Solid Edge part; units mm, degrees
sketch "Sketch1" plane through (0, 0, 0) normal (0, -1, 0) x (1, 0, 0)
  line L0 (0, 0) -> (0, -330.2)
  line L1 (0, 0) -> (0, 330.2)
  arc A0 (0, 330.2) -> (0, -330.2) centre (0, 0) cw
revolve "RevolvedProtrusion1" add sketch "Sketch1" angle 360 about axis through (0, 0, 0) along (0, 0, 1)
sketch "Sketch2" plane through (0, 0, 0) normal (0, -1, 0) x (1, 0, 0)
  line L0 (0, -305.264) -> (125.8807, -305.264)
revolve "RevolvedCutout1" cut sketch "Sketch2" angle 360 about axis through (0, 0, -305.264) along (0, 0, -1) material side at (62.9404, 0, -305.314)
sketch "Sketch3" plane through (0, 0, 0) normal (0, -1, 0) x (1, 0, 0)
  line L0 (0, -76.2) -> (330.2, -76.2)
  line L1 (330.2, 0) -> (330.2, -76.2)
  line L2 (0, 0) -> (330.2, 0)
  line L3 (0, 0) -> (0, -76.2)
revolve "RevolvedProtrusion2" add sketch "Sketch3" angle 360 about axis through (0, 0, 0) along (0, 0, -1)
sketch "Sketch4" plane through (0, 0, 330.2) normal (0, 0, 1) x (1, 0, 0)
  circle A0 centre (0, 0) radius 25.4
extrude "Protrusion1" add sketch "Sketch4" against normal up to vertex (330.2 mm away) and the other way blind 25.4
shell "Thinwall_1" thickness 6.35 removed faces 1 at (-17.4413, -16.4253, 355.6)
sketch "Sketch5" plane through (0, 0, 355.6) normal (0, 0, 1) x (0, -1, 0)
  circle A0 centre (0, 0) radius 19.05
  circle A1 centre (0, 0) radius 6.35
extrude "ExtrudedProtrusion_3" add sketch "Sketch5" against normal blind 6.35
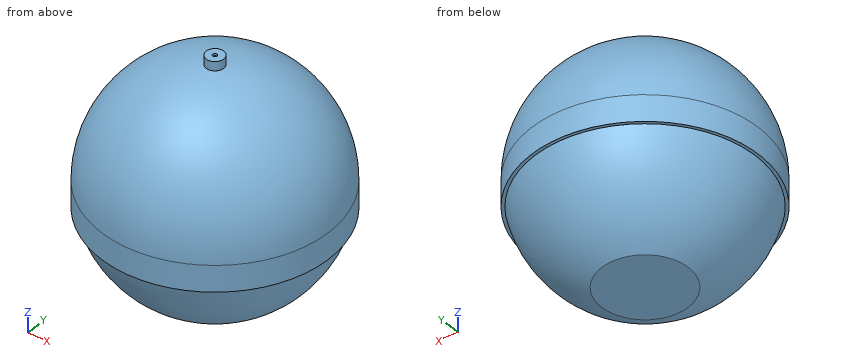
Source: CAD feature listing. Evaluate the final solid. Frame: model axes, mm. Give positions to 0.01 mm unless a question says otherwise; leave off trailing zeros. Write each loop counter-clockwise with the first axis right and the second up, starting at its lowest first coordinate (ties: lowest second). Pieces come first, ordered by that corner, then holes. Notation, with made-up numbers: (35.25, 67.5) - (72.25, 67.5) arc R21 cw to (72.25, 99.5) - close; hole circle Ø8 at (-17.5, -39). An arc over 180 degrees is marked (long way). One line per item, written item: value. Start each with the question number.
Q1. Section query D-D, the plane y = -112.5. Return the cut outline in (x, z), then the cut area to 3 significant figures.
Q2. Section query A-A, the plane y = 277. Return the cut outline in (x, z), then the cut area to 3 significant figures.
Q3. First-contact query: pin 1 Ø4 at (x, y) = (-200.5, 0) entering from -Z; pin 2 Ø6 at (y, z) = (-13.5, -40.5) entering from +X; pin 3 Ø2 at (y, z) = (-105.5, 99.5) entering from +X. Flat tips, straight axial feed; report the tip coordinate or a pass-through.
Q4. Material intervals for probe 1 along Y at (x, z) = (0, 331); probe 2 along X at (y, z) = (129.5, 67.5); probe 3 along X at (y, z) = (-111, -8), sorted ascending. Write a range as from..to.
Q5. Section query B-B, the plane x = -286.5. Return the cut outline in (y, z).
Q6. Section query C-C, the plane z = -46.5. Return the cut outline in (x, y).
Answer:
1. outline: (-310.44, -76.2) - (-300.95, -76.2) arc R310.44 ccw to (-56.48, -305.26) - (56.48, -305.26) arc R310.44 ccw to (300.95, -76.2) - (310.44, -76.2) - (310.44, 0) arc R310.44 ccw to (-310.44, 0) - close; hole (-303.68, -69.85) - (-295.54, -69.85) arc R303.68 ccw to (-53.6, -298.91) - (53.6, -298.91) arc R303.68 ccw to (295.54, -69.85) - (303.68, -69.85) - (303.68, 0) arc R303.68 ccw to (-303.68, 0) - close
1. area: 13,100 mm2
2. outline: (-179.73, -76.2) - (-162.78, -76.2) arc R179.73 ccw to (162.78, -76.2) - (179.73, -76.2) - (179.73, 0) arc R179.73 ccw to (-179.73, 0) - close; hole (-167.78, -69.85) - (-152.55, -69.85) arc R167.78 ccw to (152.55, -69.85) - (167.78, -69.85) - (167.78, 0) arc R167.78 ccw to (-167.78, 0) - close
2. area: 13,200 mm2
3. pin 1: stops at z = -263.87
3. pin 2: stops at x = 330.03
3. pin 3: stops at x = 297.14
4. probe 1: y = -25.4..-19.05, 19.05..25.4
4. probe 2: x = -296.15..-289.05, 289.05..296.15
4. probe 3: x = -310.98..-304.23, 304.23..310.98
5. outline: (-164.16, -76.2) - (-145.41, -76.2) arc R164.16 ccw to (145.41, -76.2) - (164.16, -76.2) - (164.16, 0) arc R164.16 ccw to (-164.16, 0) - close; hole (-150.99, -69.85) - (-133.86, -69.85) arc R150.99 ccw to (133.86, -69.85) - (150.99, -69.85) - (150.99, 0) arc R150.99 ccw to (-150.99, 0) - close
6. outline: circle Ø660.4 at (0, 0); hole circle Ø647.7 at (0, 0)
